Check sheet for the modelled part. Datum: model origin and axes. Units: mm. Give positions to 0.01 mm unless a question says otherwise; leave off trailing zeros. Loops run counter-clockwise (first coordinate to the right, second up) from the corner with the lowest first, then second, coordinate; pieces in that order, holes last. Notation, with made-up numbers: (77, 81) - (130, 81) arc R11 cw to (130, 97) - close; hole circle Ø5 at (21, 54). An arc over 180 degrees is marked (long way). Answer in a Markdown table with one row per item. Add a question column.
(1) Sectioned sample at B-B on x = 1. Enter the section's corners in (y, z), then the cut area to 3 significant figures.
(2) Sectioned sample at A-A on y = -80. Enter the section's corners in (x, z), then the cut area to 3 significant figures.
(3) Sectioned sample at D-D on x = -22. Enter the section's corners in (y, z), then the cut area to 3 significant figures.
(4) Thickness scan on L1, parallel to X at y = 65.5, z = 0.7; L2, parallel to X at y = -5.5, z = 0.6; L3, parallel to X at y = -8, z = 0.3. Record the ranges inside material, lowest first.
(5) Go/stop test with flat-tipped pins: P1, Ø1.5, axis at x = -47.5, z = 1.5, coming from the +Y side; P2, Ø0.9, axis at x = -46, z = 2, coming from the -Y side; P3, Ø0.9, axis at x = -49, z = 1, coming from the -Y side. Record where each tip stops, or that it passes through.
(6) Sectioned sample at C-C on y = 33. Enter the section's corners in (x, z), then the cut area to 3 significant figures.
from build123d import *

# Parameters (mm, degrees)
F0_W     = 90
F0_H     = 227
F1_DEPTH = 3
F3_DEPTH = 3


# Not quite as in the source:
# - a feature names something its author has since deleted; it is built from what else it names


with BuildPart() as f1:
    # F0 (on Top) → F1 (new body)
    with BuildSketch(Plane.XY):
        Rectangle(F0_W, F0_H)
        with BuildLine():
            ThreePointArc((-30.2779513906, -108.4999991059), (-34.4140194322, -106.3094369778), (-34.9259618692, -101.6571755682))
            Line((-34.9259618692, -101.6571755682), (-3.7184084714, -22.9447908871))
            ThreePointArc((-3.7184084714, -22.9447908871), (-8.85e-08, -20.4190497173), (3.7184082943, -22.9447908871))
            Line((3.7184082943, -22.9447908871), (34.9259616921, -101.6571755682))
            ThreePointArc((34.9259616921, -101.6571755682), (34.4140192551, -106.3094369778), (30.2779512136, -108.4999991059))
            Line((30.2779512136, -108.4999991059), (-30.2779513906, -108.4999991059))
        make_face(mode=Mode.SUBTRACT)
        with BuildLine():
            ThreePointArc((-40, 61.145500066), (-35.9380691891, 66.0567143962), (-30.3519895215, 62.9883236038))
            Line((-30.3519895215, 62.9883236038), (-6.4745976856, 2.7642353066))
            ThreePointArc((-6.4745976856, 2.7642353066), (-5.9466134034, 0), (-6.4745976856, -2.7642353066))
            Line((-6.4745976856, -2.7642353066), (-30.3519895215, -62.9883236038))
            ThreePointArc((-30.3519895214, -62.9883236038), (-35.9380691891, -66.0567143962), (-40, -61.145500066))
            Line((-40, -61.145500066), (-40, 61.145500066))
        make_face(mode=Mode.SUBTRACT)
        with BuildLine():
            ThreePointArc((30.2779512136, 108.4999991059), (34.4140192551, 106.3094369778), (34.9259616921, 101.6571755682))
            Line((34.9259616921, 101.6571755682), (3.7184082943, 22.9447908871))
            ThreePointArc((3.7184082943, 22.9447908871), (-8.85e-08, 20.4190497173), (-3.7184084714, 22.9447908871))
            Line((-3.7184084714, 22.9447908871), (-34.9259618692, 101.6571755682))
            ThreePointArc((-34.9259618692, 101.6571755682), (-34.4140194322, 106.3094369778), (-30.2779513906, 108.4999991059))
            Line((-30.2779513906, 108.4999991059), (30.2779512136, 108.4999991059))
        make_face(mode=Mode.SUBTRACT)
        with BuildLine():
            Line((6.4745976856, 2.7642353066), (30.3519895215, 62.9883236038))
            ThreePointArc((30.3519895215, 62.9883236038), (35.9380691891, 66.0567143962), (40, 61.145500066))
            Line((40, 61.145500066), (40, -61.145500066))
            ThreePointArc((40, -61.145500066), (35.9380691891, -66.0567143962), (30.3519895214, -62.9883236038))
            Line((30.3519895215, -62.9883236038), (6.4745976856, -2.7642353066))
            ThreePointArc((6.4745976856, -2.7642353066), (5.9466134034, 0), (6.4745976856, 2.7642353066))
        make_face(mode=Mode.SUBTRACT)
    extrude(amount=F1_DEPTH)

    # F2 (on face) → F3 (join, through all)
    with BuildSketch(Plane.XY.offset(3)):
        Polygon((-45, 95.5), (-45, 107.5), (-51, 107.5), (-51, 92.5), (-48, 92.5), (-48, 95.5), align=None)
        Polygon((51, 107.5), (45, 107.5), (45, 95.5), (48, 95.5), (48, 92.5), (51, 92.5), align=None)
        Polygon((-45, 45.5), (-45, 57.5), (-51, 57.5), (-51, 42.5), (-48, 42.5), (-48, 45.5), align=None)
        Polygon((51, 57.5), (45, 57.5), (45, 45.5), (48, 45.5), (48, 42.5), (51, 42.5), align=None)
        Polygon((-45, 113.5), (-45, 107.5), (-45, 95.5), (-45, 57.5), (-45, 45.5), (-45, 7.5), (-45, -4.5), (-45, -42.5), (-45, -54.5), (-45, -92.5), (-45, -104.5), (-45, -113.5), (45, -113.5), (45, -104.5), (45, -92.5), (45, -54.5), (45, -42.5), (45, -4.5), (45, 7.5), (45, 45.5), (45, 57.5), (45, 95.5), (45, 107.5), (45, 113.5), align=None)
        with BuildLine():
            Line((3.7184082943, -22.9447908871), (34.9259616921, -101.6571755682))
            ThreePointArc((34.9259616921, -101.6571755682), (34.4140192551, -106.3094369778), (30.2779512136, -108.4999991059))
            Line((30.2779512136, -108.4999991059), (-30.2779513906, -108.4999991059))
            ThreePointArc((-30.2779513906, -108.4999991059), (-34.4140194322, -106.3094369778), (-34.9259618692, -101.6571755682))
            Line((-34.9259618692, -101.6571755682), (-3.7184084714, -22.9447908871))
            ThreePointArc((-3.7184084714, -22.9447908871), (-8.85e-08, -20.4190497173), (3.7184082943, -22.9447908871))
        make_face(mode=Mode.SUBTRACT)
        with BuildLine():
            ThreePointArc((-30.3519895214, -62.9883236038), (-35.9380691891, -66.0567143962), (-40, -61.145500066))
            Line((-40, -61.145500066), (-40, 61.145500066))
            ThreePointArc((-40, 61.145500066), (-35.9380691891, 66.0567143962), (-30.3519895215, 62.9883236038))
            Line((-30.3519895215, 62.9883236038), (-6.4745976856, 2.7642353066))
            ThreePointArc((-6.4745976856, 2.7642353066), (-5.9466134034, 0), (-6.4745976856, -2.7642353066))
            Line((-6.4745976856, -2.7642353066), (-30.3519895215, -62.9883236038))
        make_face(mode=Mode.SUBTRACT)
        with BuildLine():
            ThreePointArc((-34.9259618692, 101.6571755682), (-34.4140194322, 106.3094369778), (-30.2779513906, 108.4999991059))
            Line((-30.2779513906, 108.4999991059), (30.2779512136, 108.4999991059))
            ThreePointArc((30.2779512136, 108.4999991059), (34.4140192551, 106.3094369778), (34.9259616921, 101.6571755682))
            Line((34.9259616921, 101.6571755682), (3.7184082943, 22.9447908871))
            ThreePointArc((3.7184082943, 22.9447908871), (-8.85e-08, 20.4190497173), (-3.7184084714, 22.9447908871))
            Line((-3.7184084714, 22.9447908871), (-34.9259618692, 101.6571755682))
        make_face(mode=Mode.SUBTRACT)
        with BuildLine():
            ThreePointArc((6.4745976856, -2.7642353066), (5.9466134034, 0), (6.4745976856, 2.7642353066))
            Line((6.4745976856, 2.7642353066), (30.3519895215, 62.9883236038))
            ThreePointArc((30.3519895215, 62.9883236038), (35.9380691891, 66.0567143962), (40, 61.145500066))
            Line((40, 61.145500066), (40, -61.145500066))
            ThreePointArc((40, -61.145500066), (35.9380691891, -66.0567143962), (30.3519895214, -62.9883236038))
            Line((30.3519895215, -62.9883236038), (6.4745976856, -2.7642353066))
        make_face(mode=Mode.SUBTRACT)
        Polygon((-45, -4.5), (-45, 7.5), (-51, 7.5), (-51, -7.5), (-48, -7.5), (-48, -4.5), align=None)
        Polygon((-45, -54.5), (-45, -42.5), (-51, -42.5), (-51, -57.5), (-48, -57.5), (-48, -54.5), align=None)
        Polygon((-45, -104.5), (-45, -92.5), (-51, -92.5), (-51, -107.5), (-48, -107.5), (-48, -104.5), align=None)
        Polygon((51, -92.5), (45, -92.5), (45, -104.5), (48, -104.5), (48, -107.5), (51, -107.5), align=None)
        Polygon((51, -42.5), (45, -42.5), (45, -54.5), (48, -54.5), (48, -57.5), (51, -57.5), align=None)
        Polygon((51, 7.5), (45, 7.5), (45, -4.5), (48, -4.5), (48, -7.5), (51, -7.5), align=None)
    extrude(amount=-F3_DEPTH)


solid = f1.part
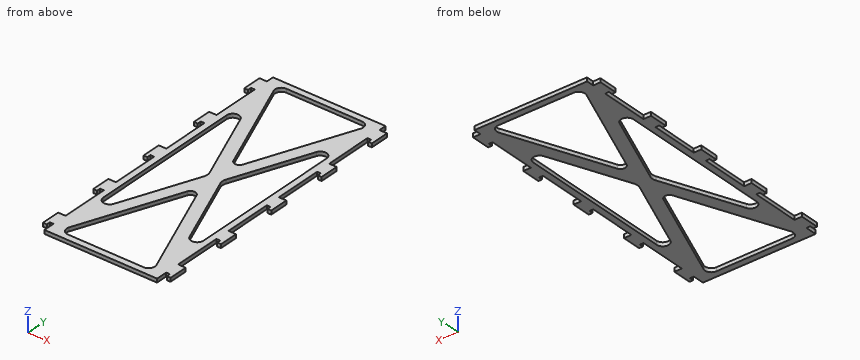
Reply:
| question | item | result |
|---|---|---|
| 1 | outline | (-113.5, 0) - (-108.5, 0) - (-108.5, 3) - (-113.5, 3) - close; (-20.55, 0) - (20.55, 0) - (20.55, 3) - (-20.55, 3) - close; (108.5, 0) - (113.5, 0) - (113.5, 3) - (108.5, 3) - close |
| 1 | area | 153 mm^2 |
| 2 | outline | (-45, 0) - (-26.34, 0) - (-26.34, 3) - (-45, 3) - close; (26.34, 0) - (45, 0) - (45, 3) - (26.34, 3) - close |
| 2 | area | 112 mm^2 |
| 3 | outline | (-113.5, 0) - (-108.5, 0) - (-108.5, 3) - (-113.5, 3) - close; (-69.06, 0) - (-41.92, 0) - (-41.92, 3) - (-69.06, 3) - close; (41.92, 0) - (69.06, 0) - (69.06, 3) - (41.92, 3) - close; (108.5, 0) - (113.5, 0) - (113.5, 3) - (108.5, 3) - close |
| 3 | area | 193 mm^2 |
| 4 | L1 | -45 to -37.46, -32.54 to -20.59, 20.59 to 32.54, 37.46 to 45 |
| 4 | L2 | -51 to -48, -45 to -40, -7.56 to 7.56, 40 to 45, 48 to 51 |
| 4 | L3 | -45 to -40, -8.55 to 8.55, 40 to 45 |
| 5 | P1 | y = 107.5 |
| 5 | P2 | y = -104.5 |
| 5 | P3 | y = -107.5 |
| 6 | outline | (-45, 0) - (-40, 0) - (-40, 3) - (-45, 3) - close; (-18.46, 0) - (-7.71, 0) - (-7.71, 3) - (-18.46, 3) - close; (7.71, 0) - (18.46, 0) - (18.46, 3) - (7.71, 3) - close; (40, 0) - (45, 0) - (45, 3) - (40, 3) - close |
| 6 | area | 94.5 mm^2 |
